Part model, mm, in its own coordinate system. Round coordinates to 2 decimals unless told otherwise and drop trailing zeros. Write each loop counter-clockwise with the first axis right and the second up, starting at its lowest first coordinate (ties: lowest second). Pieces come first, ordered by that corner, then holes. Notation, with made-up numbers: (18.25, -5) -> (25.25, -5) arc R25 ccw to (25.25, 17) -> close; hole circle Ø9 at (-35, -20). An arc over 180 degrees is marked (long way). Use CSV: the item, a comma, the result in double quotes. Start each with the question number.
```python
from build123d import *

# Parameters (mm, degrees)
SCHIZZO1_R                   = 12.7
ESTRUSIONE_ESTRUSIONE1_DEPTH = 3.81
SCHIZZO2_R                   = 6.35
ESTRUSIONE_ESTRUSIONE2_DEPTH = 15.24
FORI_ALESATO_4_0MM1_D        = 6.35
FORO_PER_VITE_M3_1_D         = 3.4
RIPETIZIONECIRCOLARE2_COUNT  = 3


with BuildPart() as part:
    # Schizzo1 → Estrusione-Estrusione1 (new body)
    with BuildSketch(Plane(origin=(0, 0, 0), x_dir=(0, 1, 0), z_dir=(0, 0, 1))):
        with Locations(Location((0, 0, 0), (0, 0, 270))):
            Circle(SCHIZZO1_R)
    extrude(amount=ESTRUSIONE_ESTRUSIONE1_DEPTH)

    # Schizzo2 → Estrusione-Estrusione2 (add)
    with BuildSketch(Plane.XY.offset(3.81)):
        Circle(SCHIZZO2_R)
    extrude(amount=ESTRUSIONE_ESTRUSIONE2_DEPTH)

    # Fori Alesato Ø4.0mm1 (through all)
    with Locations(Plane.XY.offset(19.05)):
        with Locations((0, 0)):
            Hole(FORI_ALESATO_4_0MM1_D / 2)

    # Foro per Vite M3-1 (through all)
    with Locations(Plane.XY.offset(3.81)):
        with Locations((0, 9.525)):
            foro_per_vite_m3_1 = Hole(FORO_PER_VITE_M3_1_D / 2)

    # RipetizioneCircolare2: Foro per Vite M3-1 ×3 about axis
    ripetizionecircolare2_axis = Axis((0, 0, 0), (0, 0, 1))
    for i in range(1, RIPETIZIONECIRCOLARE2_COUNT):
        add(foro_per_vite_m3_1.rotate(ripetizionecircolare2_axis, i * 360 / RIPETIZIONECIRCOLARE2_COUNT), mode=Mode.SUBTRACT)


solid = part.part
```
1. Band-saw the part on C-C (y = -5). List the corners of the cut face in (x, z).
2. Drill centre lines: line 1 along Y through (x, z) = (0, 2.55) (3 decimals); line 2 along Y through (x, z) = (0, 10.75) (3 decimals); line 3 along Z through (x, y) = (-8, -3). Where is each one in solid material? Low to high. Write a range as [from, to].
3. Band-saw the part on D-D (z = 11). List the corners of the cut face in (x, y) (3 decimals).
4. Band-saw the part on B-B (x = 0). List the corners of the cut face in (y, z) (3 decimals).
5. Flat gauge pins, fed straight in: pin 1 (2.5 mm diameter, centred on x = 0, y = 9.525, fed in from +Z); pin 2 (2 mm diameter, centred on x = 0.5, z = 16.5, fed in from -Y); pin 3 (2 mm diameter, centred on x = 3.5, z = 10.5, fed in from -Y). Where does each tip first touch, or does it go through?
6. Pull direction X, two halves, no side cores. Call faces 1 (the cylindrical face through (-1.38, -6.2, 11.32)), 2 (the cylindrical face through (-7.88, -6.42, 1.88)), 3 (the flat face through (3, 6, 3.81)), 4 (the cylindrical face through (6.679, -5.414, 1.878)): released by +X, released by -X, zero draft, split by the parting line, or undercut.
7. Band-saw the part on A-A (y = 0). List the corners of the cut face in (x, z) (3 decimals).
Answers below:
1,outline,"(-11.67, 0) -> (-9.93, 0) -> (-9.93, 3.81) -> (-11.67, 3.81) -> close; (-6.57, 0) -> (6.57, 0) -> (6.57, 3.81) -> (3.91, 3.81) -> (3.91, 19.05) -> (-3.91, 19.05) -> (-3.91, 3.81) -> (-6.57, 3.81) -> close; (9.93, 0) -> (11.67, 0) -> (11.67, 3.81) -> (9.93, 3.81) -> close"
2,line 1,"y = [-12.7, -3.175], [3.175, 7.825], [11.225, 12.7]"
2,line 2,"y = [-6.35, -3.175], [3.175, 6.35]"
2,line 3,"z = [0, 3.81]"
3,outline,"circle Ø12.7 at (0, 0); hole circle Ø6.35 at (0, 0)"
4,outline,"(-12.7, 0) -> (-3.175, 0) -> (-3.175, 19.05) -> (-6.35, 19.05) -> (-6.35, 3.81) -> (-12.7, 3.81) -> close; (3.175, 0) -> (7.825, 0) -> (7.825, 3.81) -> (6.35, 3.81) -> (6.35, 19.05) -> (3.175, 19.05) -> close; (11.225, 0) -> (12.7, 0) -> (12.7, 3.81) -> (11.225, 3.81) -> close"
5,pin 1,"passes through"
5,pin 2,"stops at y = -6.35"
5,pin 3,"stops at y = -5.84"
6,face 1,"split by the parting line"
6,face 2,"undercut"
6,face 3,"zero draft"
6,face 4,"undercut"
7,outline,"(-12.7, 0) -> (-3.175, 0) -> (-3.175, 19.05) -> (-6.35, 19.05) -> (-6.35, 3.81) -> (-12.7, 3.81) -> close; (3.175, 0) -> (12.7, 0) -> (12.7, 3.81) -> (6.35, 3.81) -> (6.35, 19.05) -> (3.175, 19.05) -> close"
